Autodesk Inventor part; units mm, degrees
ref_plane "YZ Plane" through (0, 0, 0) normal (1, 0, 0) x (0, 1, 0)
ref_plane "XZ Plane" through (0, 0, 0) normal (0, 1, 0) x (-1, 0, 0)
ref_plane "XY Plane" through (0, 0, 0) normal (0, 0, 1) x (1, 0, 0)
sketch "Sketch1" plane through (0, 0, 0) normal (0, 0, 1) x (1, 0, 0)
  circle A0 centre (0, 0) radius 30
  dimension "d0" = 60
extrude "Initial Cylinder" add sketch "Sketch1" along normal blind 4.78
sketch "Sketch2" plane through (0, 0, 4.78) normal (0, 0, 1) x (1, 0, 0)
  circle A0 centre (0, 0) radius 16
  dimension "d3" = 32
extrude "Through-hole" cut sketch "Sketch2" against normal blind 548
sketch "Sketch3" plane through (0, 0, 4.78) normal (0, 0, 1) x (1, 0, 0)
  circle A0 centre (0, 0) radius 29.25
  dimension "d6" = 58.5
extrude "snug ring fit" cut sketch "Sketch3" against normal blind 4
sketch "Sketch5" plane through (0, 0, 0) normal (0, 1, 0) x (-1, 0, 0)
  line L0 (30, 4.78) -> (-30, 4.78)
  line L1 (30, 0) -> (-30, 0)
  point P0 (0, 0)
  dimension "d16" = 4.78
sketch "Sketch6" plane through (0, 0, 0.78) normal (0, 0, 1) x (1, 0, 0)
  circle A0 centre (0, 0) radius 17.65
  dimension "d17" = 35.3
extrude "Piezo Puzzle indent" cut sketch "Sketch6" against normal blind 0.5
sketch "Sketch7" plane through (0, 0, 0) normal (0, 0, -1) x (-1, 0, 0)
  circle A0 centre (0, 0) radius 16
  circle A1 centre (0, 0) radius 30
extrude "Extra forward thickness" add sketch "Sketch7" along normal blind 1
sketch "Sketch8" plane through (0, 0, 0.28) normal (0, 0, 1) x (1, 0, 0)
  circle A0 centre (0, 0) radius 16
  circle A1 centre (0, 0) radius 17.65
  circle A2 centre (0, 0) radius 17.75
  dimension "d26" = 35.5
extrude "Piezo accomodation for EFT^" cut sketch "Sketch8" along normal mid plane 1 contours A0 | A1 | A2
sketch "Sketch9" plane through (0, 0, 4.78) normal (0, 0, 1) x (1, 0, 0)
  circle A0 centre (0, 0) radius 29.25
  circle A1 centre (0, 0) radius 30
extrude "Downoward extension" add sketch "Sketch9" along normal blind 14
sketch "Sketch4" plane through (0, 0, 0) normal (0, 1, 0) x (-1, 0, 0)
  line L0 (30, 4.78) -> (-30, 4.78)
  line L1 (0, 4.78) -> (0, 5.78)
  circle A0 centre (0, 5.78) radius 2.825
  point P0 (0, 0)
  dimension "d10" = 5.65
  dimension "d29" = 1
extrude "Bolt through-hole" cut sketch "Sketch4" along normal mid plane 548
sketch "Sketch11" plane through (0, 0, 18.78) normal (0, 0, 1) x (1, 0, 0)
  line L0 (0, 0) -> (-30, 0)
  circle A0 centre (0, 0) radius 30
  line L1 (-27.0677, -7) -> (-27.0677, 7)
  line L2 (-27.0677, 7) -> (-32.9323, 7)
  line L3 (-32.9323, 7) -> (-32.9323, -7)
  line L4 (-32.9323, -7) -> (-27.0677, -7)
  line L5 (-27.0677, -7) -> (-32.9323, 7) construction
  line L6 (-27.0677, 7) -> (-32.9323, -7) construction
  point P0 (-29.1719, 7)
  point P1 (-29.1719, -7)
  dimension "d32" = 14
extrude "Extrusion10" cut sketch "Sketch11" against normal blind 7 contours L1 L4 A0 L0 | L0 A0 L2 L1
properties part number "Diaphragm_lock"
Can you work these out from the model? Positions are in its coordinate system, mm. A direction names the side the tool comes from. Round coordinates to 2 decimals unless told otherwise and drop trailing zeros. Order: outer loops, then holes, each group sorted by start corner. A loop starts at its lowest first (then second) coordinate and runs counter-clockwise, first axis right, second up. Notation, with made-up numbers: (4, 52.25) - (19, 52.25) arc R25 cw to (19, 82.25) - close; hole circle Ø11 at (36.25, 15). An arc over 180 degrees is marked (long way). Answer in a Markdown table with one row per item.
(1) Suppose I cut it at B-B, the plane y = 0. Please give me the cut outline in (x, z), plus the area to 3 significant figures.
From the geometry:
| item | result |
|---|---|
| outline | (-30, -1) - (-16, -1) - (-16, -0.22) - (-17.75, -0.22) - (-17.75, 0.78) - (-29.25, 0.78) - (-29.25, 11.78) - (-30, 11.78) - close; (16, -1) - (30, -1) - (30, 18.78) - (29.25, 18.78) - (29.25, 0.78) - (17.75, 0.78) - (17.75, -0.22) - (16, -0.22) - close |
| area | 68.1 mm2 |
(2) Suppose I cut it at C-C, the plane z = 5.78. Please give me the cut outline in (x, y) (3 decimals).
From the geometry:
| item | result |
|---|---|
| outline | (-2.825, -29.867) - (-2.825, -29.113) arc R29.25 cw to (-2.825, 29.113) - (-2.825, 29.867) arc R30 ccw to start; (2.825, -29.867) arc R30 ccw to (2.825, 29.867) - (2.825, 29.113) arc R29.25 cw to (2.825, -29.113) - close |
(3) Suppose I cut it at D-D, the plane x = 8. Please give me the cut outline in (y, z).
From the geometry:
| item | result |
|---|---|
| outline | (-28.91, -1) - (-13.86, -1) - (-13.86, -0.22) - (-15.84, -0.22) - (-15.84, 0.78) - (-28.13, 0.78) - (-28.13, 18.78) - (-28.91, 18.78) - close; (13.86, -1) - (28.91, -1) - (28.91, 18.78) - (28.13, 18.78) - (28.13, 0.78) - (15.84, 0.78) - (15.84, -0.22) - (13.86, -0.22) - close |
(4) Suppose I cut it at A-A, the plane x = 0. Please give me the cut outline in (y, z) (3 decimals).
From the geometry:
| item | result |
|---|---|
| outline | (-30, -1) - (-16, -1) - (-16, -0.22) - (-17.75, -0.22) - (-17.75, 0.78) - (-29.25, 0.78) - (-29.25, 2.955) - (-30, 2.955) - close; (-30, 8.605) - (-29.25, 8.605) - (-29.25, 18.78) - (-30, 18.78) - close; (16, -1) - (30, -1) - (30, 2.955) - (29.25, 2.955) - (29.25, 0.78) - (17.75, 0.78) - (17.75, -0.22) - (16, -0.22) - close; (29.25, 8.605) - (30, 8.605) - (30, 18.78) - (29.25, 18.78) - close |
(5) If we mould it in two halves opening along Y, with no side actions, what happens to faces 3 (the face through (-1.3, 29.56, 3.27)), 4 (the face through (-29.4, 0.1, 11.78))? For each: released by +Y, released by -Y, zero draft, split by the parting line, or undercut.
From the geometry:
| item | result |
|---|---|
| face 3 | zero draft |
| face 4 | undercut |
(6) For P1, Ø5, axis at x = -8.5, z = 12, coming from the +Y side; P2, Ø1.5, axis at x = -9.5, z = 5, coming from the -Y side; P3, Ø1.8, axis at x = -29, y = 1, coming from the +Z side, each with a flat end and sliding along its axis, tell me the tip position at first contact or that it passes through.
From the geometry:
| item | result |
|---|---|
| P1 | stops at y = 29.39 |
| P2 | stops at y = -28.7 |
| P3 | stops at z = 11.78 |
(7) Please list where these lines run through material, in increasing order: L1, parallel to X at y = 0, z = 3.35; L2, parallel to Y at x = 0, z = 0.05; L3, parallel to Z at x = 0, y = 29.4 (3 decimals). Write a range as from..to.
From the geometry:
| item | result |
|---|---|
| L1 | x = -30..-29.25, 29.25..30 |
| L2 | y = -30..-17.75, 17.75..30 |
| L3 | z = -1..2.955, 8.605..18.78 |
(8) Which directions (+Z, -Z, +X, -X, +Y, -Y) give clear straight access to the entire face, cutting with the end or side of a thin tool? Please do faces 1 (the face through (-3, 16, -0.22)), 2 (the face through (-13, -13, -1)).
From the geometry:
| item | result |
|---|---|
| face 1 | +Z |
| face 2 | -Z, +X, -X, +Y, -Y |
